Can you work these out from the model? Positions are in its coordinate system, mm. Coordinates: 2 decimals unless noted, no trailing zeros. Order: outer loops, then holes, each group sorted by start corner. A loop starts at its lowest first (then second) coordinate and runs counter-clockwise, first axis right, second up. Notation, with made-up numbers: (-1.75, -11) -> (32.25, -11) arc R27 cw to (32.25, 19) -> close; hole circle Ø8 at (-24, 6). An arc over 180 degrees is marked (long way). Write item = value, one per line.
```python
from build123d import *

# Parameters (mm, degrees)
F0_R     = 2.0066
F1_DEPTH = 203.2
F2_SIZE  = 0.254
F3_D     = 3.175
F3_DEPTH = 5.207
F3_TIP   = 0.9538662327


with BuildPart() as f1:
    # F0 (on Top) → F1 (new body)
    with BuildSketch(Plane.XY):
        Circle(F0_R)
    extrude(amount=F1_DEPTH)

    # F2
    f2_edges = [f1.edges().sort_by_distance(p)[0] for p in [
        (-2.0066, 0, 0),
        (-2.0066, 0, 203.2),
    ]]
    chamfer(f2_edges, length=F2_SIZE)

    # F3
    with Locations(Plane(origin=(0, 0, 0), x_dir=(1, 0, 0), z_dir=(0, 0, -1))):
        with Locations((0, 0)):
            Hole(F3_D / 2, depth=F3_DEPTH)
            with Locations((0, 0, -(F3_DEPTH + F3_TIP / 2))):  # 118° drill point
                Cone(0, F3_D / 2, F3_TIP, mode=Mode.SUBTRACT)


solid = f1.part
```
Item 1: I want a section at A-A, the plane z = 154.5. Please give me the cut outline in (x, y).
A:
outline = circle Ø4.01 at (0, 0)
Item 2: I'm going to push a flat-ended pin straight in: P1, Ø2, axis at x = -1.5, z = 23, coming from the -Y side. Where does the tip first touch, or does it pass through?
A:
P1 = -1.94
Item 3: If we mould it in two halves opening along Y, with no side actions, what happens to faces 1 (the flat face through (0, 0, 203.2)), 2 (the cylindrical face through (-1.479, 1.356, 100.181)), 3 (the cylindrical face through (0.34, 1.55, 2.64))? For each: pulls with the +Y half, pulls with the -Y half, needs draft (parallel to the pull), parting line crosses it, or undercut.
A:
face_1 = needs draft
face_2 = parting line crosses it
face_3 = undercut
Item 4: If I drill on probe 1 along Y at (x, z) = (0, 1.4); probe 2 along Z at (x, y) = (-0.75, -1.35); probe 3 along X at (y, z) = (-0.1, 55.5), over which ranges is the centre line in solid material (lowest first)?
A:
probe_1 = -2.01 to -1.59, 1.59 to 2.01
probe_2 = 5.23 to 203.2
probe_3 = -2 to 2
